from build123d import *

# Parameters (mm, degrees)
SKETCH_1_R           = 13
EXTRUDE_591_DEPTH    = 11.5
EXTRUDE_7_DEPTH      = 79
EXTRUDE_7_DEPTH_BACK = 11.5
SKETCH_2_W           = 1329
SKETCH_2_H           = 11.5
EXTRUDE_9_DEPTH      = 67.5
EXTRUDE_9_DEPTH_BACK = 11.5
SKETCH_3_W           = 1760
SKETCH_3_H           = 11.5
SKETCH_4_W           = 140
SKETCH_4_H           = 50
EXTRUDE_10_DEPTH     = 11.5
SKETCH_6_R           = 13
CUT_EXTRUDE_1_DEPTH  = 931.962002447


with BuildPart() as part:
    # 草图1 → Extrude 591 (new body)
    with BuildSketch(Plane.XY):
        Polygon((-744.5, 139.25), (-664.5, 59.25), (664.5, 59.25), (744.5, 139.25), (824.5, 139.25), (824.5, -139.25), (-824.5, -139.25), (-824.5, 139.25), align=None)
        with Locations((-784.5, 99.25)):
            Circle(SKETCH_1_R, mode=Mode.SUBTRACT)
        with Locations((-784.5, 19.25)):
            Circle(SKETCH_1_R, mode=Mode.SUBTRACT)
        with Locations((-784.5, -60.75)):
            Circle(SKETCH_1_R, mode=Mode.SUBTRACT)
        with Locations(Location((784.5, -60.75, 0), (0, 0, 180))):
            Circle(SKETCH_1_R, mode=Mode.SUBTRACT)
        with Locations(Location((784.5, 19.25, 0), (0, 0, 180))):
            Circle(SKETCH_1_R, mode=Mode.SUBTRACT)
        with Locations(Location((784.5, 99.25, 0), (0, 0, 180))):
            Circle(SKETCH_1_R, mode=Mode.SUBTRACT)
    extrude(amount=EXTRUDE_591_DEPTH)

    # 草图2 → 凸台-拉伸7 (add, two sides: drawn at the far end of the back side and taken through both)
    with BuildSketch(Plane.XY.offset(11.5).offset(-EXTRUDE_7_DEPTH_BACK)):
        with Locations((0, 65)):
            Rectangle(SKETCH_2_W, SKETCH_2_H)
    extrude(amount=EXTRUDE_7_DEPTH + EXTRUDE_7_DEPTH_BACK)

    # 草图3 → 凸台-拉伸9 (add, two sides: drawn at the far end of the back side and taken through both)
    with BuildSketch(Plane.XY.offset(11.5).offset(-EXTRUDE_9_DEPTH_BACK)):
        with Locations((0, -145)):
            Rectangle(SKETCH_3_W, SKETCH_3_H)
    extrude(amount=EXTRUDE_9_DEPTH + EXTRUDE_9_DEPTH_BACK)

    # 草图4 → 凸台-拉伸10 (add)
    with BuildSketch(Plane(origin=(0, -139.25, 0), x_dir=(-1, 0, 0), z_dir=(0, 1, 0))):
        with Locations((-790, 48)):
            Rectangle(SKETCH_4_W, SKETCH_4_H)
        with Locations((790, 48)):
            Rectangle(SKETCH_4_W, SKETCH_4_H)
    extrude(amount=EXTRUDE_10_DEPTH)

    # 草图6 → 切除-拉伸1 (cut, through all)
    with BuildSketch(Plane.XZ.offset(150.75)):
        with Locations((-840, 48)):
            Circle(SKETCH_6_R)
        with Locations((-760, 48)):
            Circle(SKETCH_6_R)
        with Locations(Location((760, 48, 0), (0, 0, 180))):
            Circle(SKETCH_6_R)
        with Locations(Location((840, 48, 0), (0, 0, 180))):
            Circle(SKETCH_6_R)
    extrude(amount=-CUT_EXTRUDE_1_DEPTH, mode=Mode.SUBTRACT)


solid = part.part
Read the model definition and answer for the solid it produces. Units are mm, in the model's axes. A direction names the side the tool comes from. Round coordinates to 2 decimals unless told otherwise and drop trailing zeros. Order: outer loops, then holes, each group sorted by start corner. A loop starts at its lowest first (then second) coordinate and runs counter-clockwise, first axis right, second up.
1) The part is cut by section A-A on x = -392.5. Write down the section's boundary in (y, z), plus the area to 3 significant figures.
2) The mould has two halves that part along Y. Classify faces 1 (the face through (12, -29, 11.5)), 2 (the face through (-12, -36, 0)), 3 (the face through (-9, 70.75, 45)): released by +Y, released by -Y, zero draft, split by the parting line, or undercut.
3) For faces 4 (the face through (791, -127.75, 48)), 5 (the face through (-12, -150.75, 39)), 6 (the face through (-705.06, 99.81, 5.67)), 7 (the face through (-9, 59.25, 50)), determine the directions among +Z, -Z, +X, -X, +Y, -Y from which every point of the face is accessible in a straight line to the end or side of a thin tool.
4) Flat-ended cylindrical pins translate along their axes: pin 1 (6 mm diameter, centred on y = 102.5, z = 12, fed in from +X); pin 2 (21 mm diameter, centred on x = -784.5, y = -60.75, fed in from +Z); pin 3 (12 mm diameter, centred on x = 65.5, z = 27.5, fed in from +Y); pin 4 (3.5 mm diameter, centred on y = 50, z = 6.5, fed in from -X). Find the tip coordinate at first contact, or state that the pin passes through.
5) Straight lines are drawn through the part: L1, parallel to X at y = -60, z = 6; L2, parallel to Y at x = -784.5, z = 4.5; L3, parallel to Y at x = 24, z = 41. For each, find the intervals that lie inside material, in ascending order.
Resolved:
1. outline: (-150.75, 0) - (70.75, 0) - (70.75, 90.5) - (59.25, 90.5) - (59.25, 11.5) - (-139.25, 11.5) - (-139.25, 79) - (-150.75, 79) - close
1. area: 4,230 mm2
2. face 1: undercut
2. face 2: zero draft
2. face 3: released by +Y
3. face 4: +Z, +X, -X, +Y
3. face 5: +Z, -Z, +X, -X, -Y
3. face 6: +Z, -Z, +Y
3. face 7: +Z, +X, -X
4. pin 1: stops at x = 824.5
4. pin 2: passes through
4. pin 3: stops at y = 70.75
4. pin 4: stops at x = -824.5
5. L1: x = -824.5 to -797.48, -771.52 to 771.52, 797.48 to 824.5
5. L2: y = -150.75 to -73.75, -47.75 to 6.25, 32.25 to 86.25, 112.25 to 139.25
5. L3: y = -150.75 to -139.25, 59.25 to 70.75
